Verification items for the finished model (mm, model axes). Face numbers are marked on the shaded views. A direction names the side the tool comes from. Round coordinates to 2 decimals unless told otherwise and drop trailing zeros. Write each loop counter-clockwise with the first axis right and the second up, starting at its lowest first coordinate (ties: lowest second). Pieces come first, ordered by that corner, then holes.
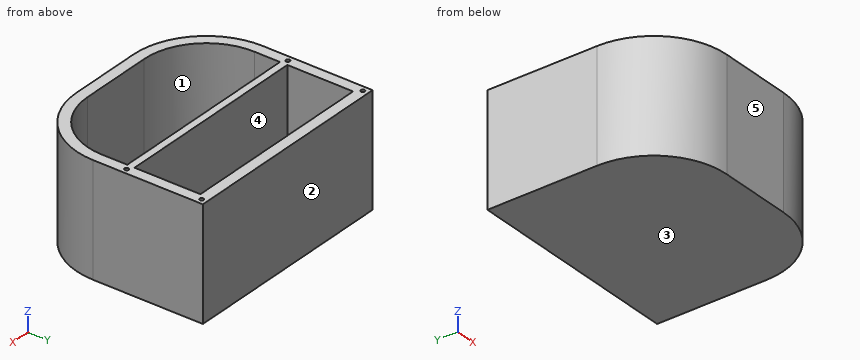
from build123d import *

# Parameters (mm, degrees)
F1_DEPTH = 7
F2_W     = 137.16
F2_H     = 5.08
F3_DEPTH = 100
F5_DEPTH = 30
F6_W     = 8
F6_H     = 8
F7_DEPTH = 25.4
F8_R     = 1.3843
F9_DEPTH = 15.24


with BuildPart() as f1:
    # F0 (on Top) → F1 (new body)
    with BuildSketch(Plane.XY):
        with BuildLine():
            Line((152.4, 0), (0, 0))
            Line((0, 0), (0, -76.2))
            ThreePointArc((0, -76.2), (14.878976, -112.121024), (50.8, -127))
            Line((50.8, -127), (101.6, -127))
            ThreePointArc((101.6, -127), (137.521024, -112.121024), (152.4, -76.2))
            Line((152.4, -76.2), (152.4, 0))
        make_face()
    extrude(amount=F1_DEPTH)

    # F2 (on face) → F3 (join)
    with BuildSketch(Plane.XY.offset(7)):
        with BuildLine():
            Line((152.4, 0), (0, 0))
            Line((0, 0), (0, -76.2))
            ThreePointArc((0, -76.2), (14.878976, -112.121024), (50.8, -127))
            Line((50.8, -127), (101.6, -127))
            ThreePointArc((101.6, -127), (137.521024, -112.121024), (152.4, -76.2))
            Line((152.4, -76.2), (152.4, 0))
        make_face()
        with BuildLine():
            Line((7.62, -53.34), (7.62, -7.62))
            Line((7.62, -7.62), (144.78, -7.62))
            Line((144.78, -7.62), (144.78, -53.34))
            Line((144.78, -53.34), (144.78, -58.42))
            Line((144.78, -58.42), (144.78, -76.2))
            ThreePointArc((144.78, -76.2), (132.132871, -106.732871), (101.6, -119.38))
            Line((101.6, -119.38), (50.8, -119.38))
            ThreePointArc((50.8, -119.38), (20.267129, -106.732871), (7.62, -76.2))
            Line((7.62, -76.2), (7.62, -58.42))
            Line((7.62, -58.42), (7.62, -53.34))
        make_face(mode=Mode.SUBTRACT)
        with Locations((76.2, -55.88)):
            Rectangle(F2_W, F2_H)
    extrude(amount=F3_DEPTH)

    # F4 (on face) → F5 (cut)
    with BuildSketch(Plane.XY.offset(107)):
        Polygon((0, 0), (0, -58.42), (0, -127), (152.4, -127), (152.4, -58.42), (152.4, 0), align=None)
    extrude(amount=-F5_DEPTH, mode=Mode.SUBTRACT)

    # F6 (on face) → F7 (cut)
    with BuildSketch(Plane.XZ.offset(58.42)):
        with Locations((11.62, 11)):
            Rectangle(F6_W, F6_H)
        with Locations((140.78, 11)):
            Rectangle(F6_W, F6_H)
    extrude(amount=-F7_DEPTH, mode=Mode.SUBTRACT)

    # F8 (on face) → F9 (cut)
    with BuildSketch(Plane.XY.offset(77)):
        with Locations((3.81, -3.81)):
            Circle(F8_R)
        with Locations((3.81, -55.88)):
            Circle(F8_R)
        with Locations((148.59, -3.81)):
            Circle(F8_R)
        with Locations((148.59, -55.88)):
            Circle(F8_R)
    extrude(amount=-F9_DEPTH, mode=Mode.SUBTRACT)


solid = f1.part
Q1. Sectioned sample at D-D (y = -47). Enter the section's corners in (x, z).
Recorded:
outline: (0, 0) - (152.4, 0) - (152.4, 77) - (144.78, 77) - (144.78, 7) - (7.62, 7) - (7.62, 77) - (0, 77) - close
Q2. Sectioned sample at B-B (x = 97.5). Enter the section's corners in (y, z).
Recorded:
outline: (-127, 0) - (0, 0) - (0, 77) - (-7.62, 77) - (-7.62, 7) - (-53.34, 7) - (-53.34, 77) - (-58.42, 77) - (-58.42, 7) - (-119.38, 7) - (-119.38, 77) - (-127, 77) - close
Q3. Release check for a two-part mould opening along Y. For the marked faces 1, 2 and 3 record: released by +Y, released by -Y, zero draft, split by the parting line, or undercut.
Recorded:
face 1: undercut
face 2: released by +Y
face 3: zero draft
Q4. Depth check by flat-ended pin: P1, Ø5, axis at x = 128.5, z = 11.5, coming from the -Y side; P2, Ø0.8, axis at x = 148.5, y = -3, coming from the +Z side; P3, Ø1, axis at y = -102.5, z = 48, coming from the -X side. Enter the tip coordinate at first touch or a pass-through.
Recorded:
P1: stops at y = -120.76
P2: stops at z = 61.76
P3: stops at x = 7.04
Q5. Sectioned sample at C-C (z = 72). Enter the section's corners in (x, y), plus the area to 3 significant figures.
Recorded:
outline: (0, -76.2) arc R50.8 ccw to (50.8, -127) - (101.6, -127) arc R50.8 ccw to (152.4, -76.2) - (152.4, 0) - (0, 0) - close; hole circle Ø2.77 at (3.81, -55.88); hole circle Ø2.77 at (3.81, -3.81); hole (7.62, -76.2) arc R43.18 ccw to (50.8, -119.38) - (101.6, -119.38) arc R43.18 ccw to (144.78, -76.2) - (144.78, -58.42) - (7.62, -58.42) - close; hole (7.62, -53.34) - (144.78, -53.34) - (144.78, -7.62) - (7.62, -7.62) - close; hole circle Ø2.77 at (148.59, -55.88); hole circle Ø2.77 at (148.59, -3.81)
area: 4,390 mm2
Q6. Sectioned sample at A-A (z = 35.5). Enter the section's corners in (x, y).
Recorded:
outline: (0, -76.2) arc R50.8 ccw to (50.8, -127) - (101.6, -127) arc R50.8 ccw to (152.4, -76.2) - (152.4, 0) - (0, 0) - close; hole (7.62, -76.2) arc R43.18 ccw to (50.8, -119.38) - (101.6, -119.38) arc R43.18 ccw to (144.78, -76.2) - (144.78, -58.42) - (7.62, -58.42) - close; hole (7.62, -53.34) - (144.78, -53.34) - (144.78, -7.62) - (7.62, -7.62) - close
Q7. Material ranges on line 1 along Y through (x, z) = (76.5, 34.5); line 2 along Y through (x, z) = (12, 44); line 3 along X through (y, z) = (-9.5, 53.5), recorded low to high.
Recorded:
line 1: y = -127 to -119.38, -58.42 to -53.34, -7.62 to 0
line 2: y = -108.99 to -95.15, -58.42 to -53.34, -7.62 to 0
line 3: x = 0 to 7.62, 144.78 to 152.4
Q8. Tool access check on the marked faces 4 and 5. Record the directions out of +Z, -Z, +X, -X, +Y, -Y that give a thin tool (end or side, any length) a straight path to the whole face; none if there is none.
Recorded:
face 4: +Z
face 5: +Z, -Z, +X, -X, -Y
